Input: part model. Units: mm. Frame: model coordinates. A direction names the side the tool comes from. Give positions to 0.01 mm unless a question says otherwise; leave off trailing zeros. Write each loop counter-clockwise with the first axis right and the second up, starting at its lowest first coordinate (ties: lowest second). Pieces come first, ordered by that corner, then holes.
```python
from build123d import *

# Parameters (mm, degrees)
BASE_FLANGE1_DEPTH = 40
CUT_EXTRUDE1_DEPTH = 649.200586239
SKETCH7_R          = 3.5
CUT_EXTRUDE2_DEPTH = 648.210166793


# Sheet-metal steps are written as plain solids
with BuildPart() as part:
    # Sketch1 → Base-Flange1 (new body)
    with BuildSketch(Plane.XY):
        with BuildLine():
            Line((0, 80), (0, 1))
            ThreePointArc((0, 1), (0.292893219, 0.292893219), (1, 0))
            Line((1, 0), (639, 0))
            ThreePointArc((639, 0), (639.707106781, 0.292893219), (640, 1))
            Line((640, 1), (640, 80))
            Line((640, 80), (641, 80))
            Line((641, 80), (641, 1))
            ThreePointArc((641, 1), (640.414213562, -0.414213562), (639, -1))
            Line((639, -1), (1, -1))
            ThreePointArc((1, -1), (-0.414213562, -0.414213562), (-1, 1))
            Line((-1, 1), (-1, 80))
            Line((-1, 80), (0, 80))
        make_face()
    extrude(amount=BASE_FLANGE1_DEPTH)

    # Sketch6 → Cut-Extrude1 (cut, through all)
    with BuildSketch(Plane(origin=(641, 0, 0), x_dir=(0, 0, -1), z_dir=(1, 0, 0))):
        with BuildLine():
            Line((-17, 70), (-17, 11))
            ThreePointArc((-17, 11), (-20, 8), (-23, 11))
            Line((-23, 11), (-23, 70))
            ThreePointArc((-23, 70), (-20, 73), (-17, 70))
        make_face()
    extrude(amount=-CUT_EXTRUDE1_DEPTH, mode=Mode.SUBTRACT)

    # Sketch7 → Cut-Extrude2 (cut, through all)
    with BuildSketch(Plane(origin=(0, 0, 0), x_dir=(1, 0, 0), z_dir=(0, 1, 0))):
        with Locations(Location((629, -20, 0), (0, 0, 270))):
            Circle(SKETCH7_R)
        with Locations(Location((629, -6, 0), (0, 0, 270))):
            Circle(SKETCH7_R)
        with Locations(Location((11, -20, 0), (0, 0, 90))):
            Circle(SKETCH7_R)
        with Locations(Location((11, -6, 0), (0, 0, 90))):
            Circle(SKETCH7_R)
        with Locations(Location((11, -34, 0), (0, 0, 270))):
            Circle(SKETCH7_R)
        with Locations(Location((629, -34, 0), (0, 0, 90))):
            Circle(SKETCH7_R)
        with Locations(Location((111, -34, 0), (0, 0, 90))):
            Circle(SKETCH7_R)
        with Locations(Location((111, -20, 0), (0, 0, 270))):
            Circle(SKETCH7_R)
        with Locations(Location((111, -6, 0), (0, 0, 270))):
            Circle(SKETCH7_R)
        with Locations(Location((529, -20, 0), (0, 0, 90))):
            Circle(SKETCH7_R)
        with Locations(Location((529, -34, 0), (0, 0, 270))):
            Circle(SKETCH7_R)
        with Locations(Location((529, -6, 0), (0, 0, 90))):
            Circle(SKETCH7_R)
    extrude(amount=-CUT_EXTRUDE2_DEPTH, mode=Mode.SUBTRACT)


solid = part.part
```
Item 1: Mould query, pull axis X, two halves, no side actions, for faces 1 (the flat face through (-1, 40, 15)), 2 (the flat face through (316, 0, 20)), 3 (the flat face through (641, 41, 15)). Classes: +X half, -X half, draft (parallel to the pull), parting line (faces both ways), or undercut.
Item 2: Section A-A (y = 21.5). Return loops of the section in (x, z), and give its area (3 significant figures).
Item 3: Ray query, line 1 (Z direction, x = 629, y = -0.5); line 2 (X direction, y = 29, z = 32); line 3 (Y direction, x = 56.5, z = 10). Return the intervals inside material, ascending.
Item 4: Set-up query: faces 4 (the flat face through (324, -1, 20)), 5 (the flat face through (640, 40, 15)). Return all of +Z, -Z, +X, -X, +Y, -Y with unobstructed straight access to the full face (end or side cutting, diameter ignored); none if empty.
Item 5: Section B-B (x = 482.5). Return loops of the section in (y, z).
Item 6: Pin query (flat end, axial travel): pin 1 (9 mm diameter, centred on x = 111, z = 34, fed in from +Y); pin 2 (6.5 mm diameter, centred on x = 111, z = 6, fed in from -Y); pin 3 (0.5 mm diameter, centred on x = 640.5, y = 49, fed in from -Z). Return the tip coordinate at first contact, or that it passes through.
Solved:
1. face 1: -X half
1. face 2: undercut
1. face 3: +X half
2. outline: (-1, 0) - (0, 0) - (0, 17) - (-1, 17) - close; (-1, 23) - (0, 23) - (0, 40) - (-1, 40) - close; (640, 0) - (641, 0) - (641, 17) - (640, 17) - close; (640, 23) - (641, 23) - (641, 40) - (640, 40) - close
2. area: 68.0 mm2
3. line 1: z = 0 to 2.5, 9.5 to 16.5, 23.5 to 30.5, 37.5 to 40
3. line 2: x = -1 to 0, 640 to 641
3. line 3: y = -1 to 0
4. face 4: +Z, -Z, +X, -X, -Y
4. face 5: +Z, -Z, +Y
5. outline: (-1, 0) - (0, 0) - (0, 40) - (-1, 40) - close
6. pin 1: stops at y = 0
6. pin 2: passes through
6. pin 3: stops at z = 0
